from build123d import *

# Parameters (mm, degrees)
BOSS_EXTRUDE1_DEPTH  = 12.5
SKETCH3_W            = 200
SKETCH3_H            = 75
BOSS_EXTRUDE2_DEPTH  = 25
BOSS_EXTRUDE3_DEPTH  = 20
MIRROR2_COPY_1_DEPTH = 20
FILLET2_R            = 15


with BuildPart() as part:
    # Sketch1 → Boss-Extrude1 (new, symmetric)
    with BuildSketch(Plane.XY):
        Polygon((0, 0), (250, 0), (250, -19.654022129), (190, -70), (150, -70), (150, -130), (190, -130), (250, -180.345977871), (250, -200), (0, -200), align=None)
        with BuildLine():
            Line((42.5, -15), (107.5, -15))
            ThreePointArc((107.5, -15), (122.5, -30), (107.5, -45))
            Line((107.5, -45), (42.5, -45))
            ThreePointArc((42.5, -45), (27.5, -30), (42.5, -15))
        make_face(mode=Mode.SUBTRACT)
        with BuildLine():
            Line((42.5, -185), (107.5, -185))
            ThreePointArc((107.5, -185), (122.5, -170), (107.5, -155))
            Line((107.5, -155), (42.5, -155))
            ThreePointArc((42.5, -155), (27.5, -170), (42.5, -185))
        make_face(mode=Mode.SUBTRACT)
    extrude(amount=BOSS_EXTRUDE1_DEPTH, both=True)

    # Sketch3 → Boss-Extrude2 (add, symmetric)
    with BuildSketch(Plane.XY):
        with Locations((75, -100)):
            Rectangle(SKETCH3_W, SKETCH3_H)
    extrude(amount=BOSS_EXTRUDE2_DEPTH, both=True)

    # Sketch4 → Boss-Extrude3 (add)
    with BuildSketch(Plane.XY.offset(12.5)):
        Polygon((250, 0), (175, 0), (175, -45), (219.793839815, -45), (250, -19.654022129), align=None)
    boss_extrude3 = extrude(amount=BOSS_EXTRUDE3_DEPTH)

    # Mirror1: Boss-Extrude3 across plane
    add(boss_extrude3.mirror(Plane.ZX.offset(-100)))

    # Mirror2: Boss-Extrude3 across plane
    add(boss_extrude3.mirror(Plane.XY))

    # Mirror2 copy 1 sketch → Mirror2 copy 1 (add)
    with BuildSketch(Plane(origin=(0, -200, -12.5), x_dir=(1, 0, 0), z_dir=(0, 0, -1))):
        Polygon((250, 0), (175, 0), (175, -45), (219.793839815, -45), (250, -19.654022129), align=None)
    extrude(amount=MIRROR2_COPY_1_DEPTH)

    # Fillet2
    fillet2_edges = [part.edges().sort_by_distance(p)[0] for p in [
        (0, 0, 0),
        (0, -200, 0),
    ]]
    fillet(fillet2_edges, radius=FILLET2_R)


solid = part.part
Geometry: final body of the model. Coordinates: model frame, mm. A direction names the side the tool comes from. Give positions to 0.01 mm unless a question says otherwise; leave off trailing zeros. Order: outer loops, then holes, each group sorted by start corner. A loop starts at its lowest first (then second) coordinate and runs counter-clockwise, first axis right, second up. Notation, with made-up numbers: (-1, 39.25) -> (5, 39.25) arc R9 ccw to (5, 54.25) -> close; hole circle Ø7 at (31.5, -29). An arc over 180 degrees is marked (long way). Answer as a JSON object with one key per item and string values.
Q1. Section A-A (x = 71). Output: boundary loops of the cut face in (y, z).
Entries:
{"outline": "(-200, -12.5) -> (-185, -12.5) -> (-185, 12.5) -> (-200, 12.5) -> close; (-155, -12.5) -> (-137.5, -12.5) -> (-137.5, -25) -> (-62.5, -25) -> (-62.5, -12.5) -> (-45, -12.5) -> (-45, 12.5) -> (-62.5, 12.5) -> (-62.5, 25) -> (-137.5, 25) -> (-137.5, 12.5) -> (-155, 12.5) -> close; (-15, -12.5) -> (0, -12.5) -> (0, 12.5) -> (-15, 12.5) -> close"}
Q2. First-contact query: pin 1 (16 mm diameter, centred on x = 200.5, z = -27, fed in from +Y); pin 2 (20 mm diameter, centred on y = -42, z = -2.5, fed in from -X); pin 3 (3 mm diameter, centred on y = -123.5, z = -14.5, fed in from +X); pin 4 (16 mm diameter, centred on y = -180, z = 25, fed in from -X). Flat tips, straight axial feed; report the tip coordinate or a pass-through.
Entries:
{"pin 1": "stops at y = 0", "pin 2": "stops at x = 0", "pin 3": "stops at x = 175", "pin 4": "stops at x = 175"}
Q3. Material intervals for probe 1 along Y at (x, z) = (78, -1.5); probe 2 along Y at (x, z) = (211, -25); probe 3 along X at (y, z) = (-64, -19), sorted ascending.
Entries:
{"probe 1": "y = -200 to -185, -155 to -45, -15 to 0", "probe 2": "y = -200 to -155, -45 to 0", "probe 3": "x = -25 to 175"}
Q4. Section B-B (y = -158.5). Output: boundary loops of the cut face in (x, z).
Entries:
{"outline": "(0, -12.5) -> (32.87, -12.5) -> (32.87, 12.5) -> (0, 12.5) -> close; (117.13, -12.5) -> (175, -12.5) -> (175, -32.5) -> (223.96, -32.5) -> (223.96, 32.5) -> (175, 32.5) -> (175, 12.5) -> (117.13, 12.5) -> close"}
Q5. Access query for faces 4 (the flat face through (175, -178, 22)), 5 (the flat face through (175, -22, -22)), 6 (the flat face through (175, -178, -22)). Directions: +Z, -Z, +X, -X, +Y, -Y. A direction counts if a zero-diameter tool reaches every point of the face in a straight line with its end or side. Return the directions, or none.
Entries:
{"face 4": "+Z, -X, -Y", "face 5": "-Z, -X, +Y", "face 6": "-Z, -X, -Y"}
Q6. Section D-D (y = -112). Output: boundary loops of the cut face in (x, z), plus the area to 3 significant figures.
Entries:
{"outline": "(-25, -25) -> (175, -25) -> (175, 25) -> (-25, 25) -> close", "area": "10,000 mm^2"}
Q7. Section C-C (x = 133). Output: boundary loops of the cut face in (y, z).
Entries:
{"outline": "(-200, -12.5) -> (-137.5, -12.5) -> (-137.5, -25) -> (-62.5, -25) -> (-62.5, -12.5) -> (0, -12.5) -> (0, 12.5) -> (-62.5, 12.5) -> (-62.5, 25) -> (-137.5, 25) -> (-137.5, 12.5) -> (-200, 12.5) -> close"}
Q8. Draft query along X for faces 1 (the flat face through (175, -22, 22)), 2 (the flat face through (75, -45, 0)), 3 (the flat face through (197, -155, -22)). Return one class per face: released by +X, released by -X, zero draft, split by the parting line, or undercut.
Entries:
{"face 1": "released by -X", "face 2": "undercut", "face 3": "zero draft"}
